```python
from build123d import *

# Parameters (mm, degrees)
SKETCH1_W               = 63.5
SKETCH1_H               = 254
BOSS_EXTRUDE1_DEPTH     = 63.5
FILLET1_RADIUS          = 31.75
FILLET1_LENGTH          = 63.5
SKETCH2_R               = 5.715
BOSS_EXTRUDE2_DEPTH     = 12.7
CUT_EXTRUDE1_DEPTH      = 84.836
CUT_EXTRUDE1_DEPTH_BACK = 60.96
SKETCH3_R               = 6.35
CUT_EXTRUDE2_DEPTH      = 69.596
CUT_EXTRUDE2_DEPTH_BACK = 117.602
SKETCH4_W               = 50.8
SKETCH4_H               = 54.314943323


with BuildPart() as part:
    # Sketch1 → Boss-Extrude1 (new body)
    with BuildSketch(Plane.XY):
        with Locations((31.75, 127)):
            Rectangle(SKETCH1_W, SKETCH1_H)
    extrude(amount=BOSS_EXTRUDE1_DEPTH)

    # Fillet1: full round fillet: the end face becomes a half cylinder, R = half its width
    fillet1_face = Plane((31.75, 0, 31.75), x_dir=(0, 0, 1), z_dir=(0, -1, 0))  # on the end face: x along it, z out of the body
    fillet1_slab = fillet1_face.offset(-FILLET1_RADIUS / 2) * Box(FILLET1_LENGTH, 2 * FILLET1_RADIUS, FILLET1_RADIUS, mode=Mode.PRIVATE)  # the body's end, R deep
    fillet1_round = Plane((31.75, 31.75, 31.75), x_dir=(0, -1, 0), z_dir=(0, 0, 1)) * Cylinder(FILLET1_RADIUS, FILLET1_LENGTH, mode=Mode.PRIVATE)  # its axis R under the face
    add(fillet1_slab - fillet1_round, mode=Mode.SUBTRACT)

    # Sketch2 → Boss-Extrude2 (add)
    with BuildSketch(Plane.XY.offset(63.5)):
        with Locations(Location((31.75, 19.05, 0), (0, 0, 180))):
            Circle(SKETCH2_R)
    boss_extrude2 = extrude(amount=BOSS_EXTRUDE2_DEPTH)

    # Mirror1: Boss-Extrude2 across plane
    add(boss_extrude2.mirror(Plane.XY.offset(31.75)))

    # Sketch3 → Cut-Extrude1 (cut, two sides: drawn at the far end of the back side and taken through both)
    with BuildSketch(Plane.XY.offset(31.75).offset(-CUT_EXTRUDE1_DEPTH_BACK)):
        with Locations(Location((31.75, 234.95, 0), (0, 0, 180))):
            Circle(SKETCH3_R)
    extrude(amount=CUT_EXTRUDE1_DEPTH + CUT_EXTRUDE1_DEPTH_BACK, mode=Mode.SUBTRACT)

    # Sketch4 → Cut-Extrude2 (cut, two sides: drawn at the far end of the back side and taken through both)
    with BuildSketch(Plane.ZY.offset(-CUT_EXTRUDE2_DEPTH_BACK)):
        with Locations((31.75, 248.137471662)):
            Rectangle(SKETCH4_W, SKETCH4_H)
    extrude(amount=CUT_EXTRUDE2_DEPTH + CUT_EXTRUDE2_DEPTH_BACK, mode=Mode.SUBTRACT)


solid = part.part
```
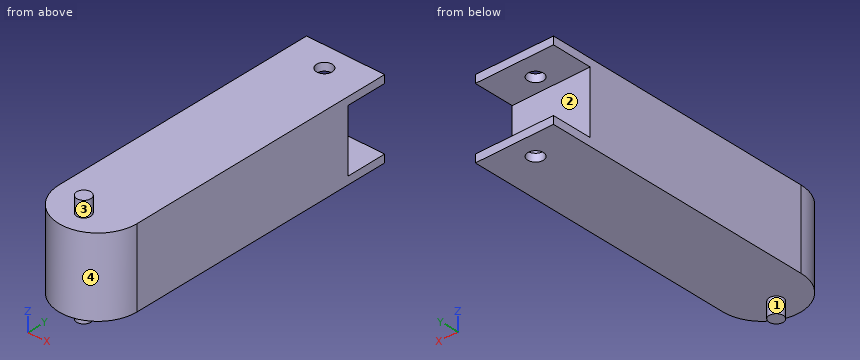
Can you work these out from the model? Positions are in its coordinate system, mm. Face numbers are marked on the shaded views. A direction names the side the tool comes from. Coordinates: 2 decimals unless noted, no trailing zeros. Order: outer loops, then holes, each group sorted by start corner. A loop starts at its lowest first (then second) coordinate and runs counter-clockwise, first axis right, second up.
1. If we section it at D-D (y = 19.05): Please give me the cut outline in (x, z) (3 decimals).
2. I need wall thicknesses on line 1 (Y direction, x = 31.75, z = 4); line 2 (Z direction, x = 45, y = 222); line 3 (X direction, y = 31, z = 56). Which ranges of each line are inside material? Lowest first, please.
3. If we section it at C-C (z = 43.5): Please give me the cut outline in (x, y).
4. If we section it at A-A (y = 234.95): Please give me the cut outline in (x, z).
5. I'm going to push flat-ended pins straight in: pin 1 (12 mm diameter, centred on x = 33, y = 93.5, fed in from +Z); pin 2 (5 mm diameter, centred on x = 43, z = 10, fed in from +Y); pin 3 (3 mm diameter, centred on x = 51, z = 29, fed in from -Y). Where does each tip first touch, or does it pass through?
6. For the marked faces 1, 2, 3 and 4, which set-ups out of +Z, -Z, +X, -X, +Y, -Y let a thin tool reach every point of the face, with its end or its side?
7. If we section it at B-B (x = 31.75): Please give me the cut outline in (y, z) (3 decimals).
Entries:
1. outline: (2.651, 0) - (26.035, 0) - (26.035, -12.7) - (37.465, -12.7) - (37.465, 0) - (60.849, 0) - (60.849, 63.5) - (37.465, 63.5) - (37.465, 76.2) - (26.035, 76.2) - (26.035, 63.5) - (2.651, 63.5) - close
2. line 1: y = 0 to 228.6, 241.3 to 254
2. line 2: z = 0 to 6.35, 57.15 to 63.5
2. line 3: x = 0.01 to 63.49
3. outline: (0, 31.75) arc R31.75 ccw to (63.5, 31.75) - (63.5, 220.98) - (0, 220.98) - close
4. outline: (0, 0) - (25.4, 0) - (25.4, 6.35) - (0, 6.35) - close; (0, 57.15) - (25.4, 57.15) - (25.4, 63.5) - (0, 63.5) - close; (38.1, 0) - (63.5, 0) - (63.5, 6.35) - (38.1, 6.35) - close; (38.1, 57.15) - (63.5, 57.15) - (63.5, 63.5) - (38.1, 63.5) - close
5. pin 1: stops at z = 63.5
5. pin 2: stops at y = 220.98
5. pin 3: stops at y = 5.43
6. face 1: -Z
6. face 2: +X, -X, +Y
6. face 3: +Z
6. face 4: +Z, -Z, -Y
7. outline: (0, 0) - (13.335, 0) - (13.335, -12.7) - (24.765, -12.7) - (24.765, 0) - (228.6, 0) - (228.6, 6.35) - (220.98, 6.35) - (220.98, 57.15) - (228.6, 57.15) - (228.6, 63.5) - (24.765, 63.5) - (24.765, 76.2) - (13.335, 76.2) - (13.335, 63.5) - (0, 63.5) - close; (241.3, 0) - (254, 0) - (254, 6.35) - (241.3, 6.35) - close; (241.3, 57.15) - (254, 57.15) - (254, 63.5) - (241.3, 63.5) - close
